```python
from build123d import *

# Parameters (mm, degrees)
SKETCH_R             = 1.6
SKETCH_R_2           = 6
PAD_DEPTH            = 4
SKETCH001_R          = 5
PAD001_DEPTH         = 12
SKETCH002_R          = 4.7
POCKET_DEPTH         = 13.001
SKETCH004_R          = 1.5
POCKET002_DEPTH      = 13.001
SKETCH005_R          = 1.5
POCKET003_DEPTH      = 4.001
POCKET003_DEPTH_BACK = 12.001
SKETCH006_R          = 4.7
SKETCH006_R_2        = 2.2
PAD002_DEPTH         = 6
SKETCH007_R          = 3
SKETCH007_R_2        = 1.5
PAD003_DEPTH         = 2
PAD003_DEPTH_BACK    = 2
SKETCH003_R          = 4.75
PAD004_DEPTH         = 2
SKETCH008_R          = 6.25
POCKET004_DEPTH      = 12.001
FILLET_R             = 1.5
FILLET001_R          = 3
FILLET002_R          = 1


with BuildPart() as part:
    # Sketch → Pad (new body)
    with BuildSketch(Plane.XY):
        Polygon((0, 20), (-26, 20), (-26, 0), (-26, -20), (0, -20), (20, -20), (20, 0), (20, 20), align=None)
        with Locations((-23, 5.9)):
            Circle(SKETCH_R, mode=Mode.SUBTRACT)
        with Locations((-23, -5.9)):
            Circle(SKETCH_R, mode=Mode.SUBTRACT)
        Circle(SKETCH_R_2, mode=Mode.SUBTRACT)
    extrude(amount=-PAD_DEPTH)

    # Sketch001 → Pad001 (join)
    with BuildSketch(Plane.XY):
        with Locations((13, -13)):
            Circle(SKETCH001_R)
        Polygon((0, 20), (20, 20), (20, 7), (0, 7), (-20, 7), (-20, 20), align=None)
    extrude(amount=PAD001_DEPTH)

    # Sketch002 (on DatumPlane) → Pocket (cut, through all)
    with BuildSketch(Plane.XZ.offset(-7)):
        with Locations((5.5, 5)):
            Circle(SKETCH002_R)
    extrude(amount=-POCKET_DEPTH, mode=Mode.SUBTRACT)

    # Sketch004 (on DatumPlane) → Pocket002 (cut, through all)
    with BuildSketch(Plane.XZ.offset(-7)):
        with Locations((-12, 5)):
            Circle(SKETCH004_R)
    extrude(amount=-POCKET002_DEPTH, mode=Mode.SUBTRACT)

    # Sketch005 → Pocket003 (cut, two sides)
    with BuildSketch(Plane.XY) as pocket003_sk:
        with Locations((13, -13)):
            Circle(SKETCH005_R)
        with Locations((13, 13)):
            Circle(SKETCH005_R)
    extrude(amount=-POCKET003_DEPTH, mode=Mode.SUBTRACT)
    extrude(pocket003_sk.sketch, amount=POCKET003_DEPTH_BACK, mode=Mode.SUBTRACT)

    # Sketch006 (on DatumPlane) → Pad002 (join)
    with BuildSketch(Plane.XZ.offset(-7)):
        with Locations((5.5, 5)):
            Circle(SKETCH006_R)
        with Locations((5.5, 5)):
            Circle(SKETCH006_R_2, mode=Mode.SUBTRACT)
    extrude(amount=-PAD002_DEPTH)

    # Sketch007 (on DatumPlane) → Pad003 (join, two sides)
    with BuildSketch(Plane.XZ.offset(-7)) as pad003_sk:
        with Locations((5.5, 5)):
            Circle(SKETCH007_R)
        with Locations((5.5, 5)):
            Circle(SKETCH007_R_2, mode=Mode.SUBTRACT)
    extrude(amount=PAD003_DEPTH)
    extrude(pad003_sk.sketch, amount=-PAD003_DEPTH_BACK)

    # Sketch003 (on DatumPlane) → Pad004 (join)
    with BuildSketch(Plane.XZ.offset(-7)):
        with BuildLine():
            ThreePointArc((-7.465411, 0), (-12, 11.75), (-16.534589, 0))
            Line((-16.534589, 0), (-7.465411, 0))
        make_face()
        with Locations((-12, 5)):
            Circle(SKETCH003_R, mode=Mode.SUBTRACT)
    extrude(amount=PAD004_DEPTH)

    # Sketch008 → Pocket004 (cut, through all)
    with BuildSketch(Plane.XY):
        Circle(SKETCH008_R)
    extrude(amount=POCKET004_DEPTH, mode=Mode.SUBTRACT)

    # Fillet
    fillet_edges = [part.edges().sort_by_distance(p)[0] for p in [
        (8, -13, 0),
    ]]
    fillet(fillet_edges, radius=FILLET_R)

    # Fillet001
    fillet001_edges = [part.edges().sort_by_distance(p)[0] for p in [
        (-26, -20, -2),
        (20, -20, -2),
        (20, 20, -2),
        (-26, 20, -2),
        (20, 7, 6),
        (-20, 20, 6),
    ]]
    fillet(fillet001_edges, radius=FILLET001_R)

    # Fillet002
    fillet002_edges = [part.edges().sort_by_distance(p)[0] for p in [
        (-20, 7, 6),
    ]]
    fillet(fillet002_edges, radius=FILLET002_R)


solid = part.part
```
Geometry: final body of the model. Coordinates: model frame, mm. A direction names the side the tool comes from. Coordinates: 2 decimals unless noted, no trailing zeros. Order: outer loops, then holes, each group sorted by start corner. A loop starts at its lowest first (then second) coordinate and runs counter-clockwise, first axis right, second up. Notation, with made-up numbers: (72.25, 38) - (119.25, 38) arc R8 cw to (119.25, 47) - close; hole circle Ø3 at (36.25, 78). An arc over 180 degrees is marked (long way). Write each question's results on one line, items separated by ' | '.
1) Section D-D, the plane x = 0. Return loops of the section in (y, z).
Results list:
outline: (-20, -4) - (-6, -4) - (-6, 0) - (-20, 0) - close; (6, -4) - (20, -4) - (20, 12) - (7, 12) - (7, 0) - (6, 0) - close
2) Section A-A, the plane x = 13. Return loops of the section in (y, z), plus the area to 3 significant figures.
Results list:
outline: (-20, -4) - (-14.5, -4) - (-14.5, 12) - (-18, 12) - (-18, 1.5) arc R1.5 cw to (-19.5, 0) - (-20, 0) - close; (-11.5, -4) - (11.5, -4) - (11.5, 12) - (7, 12) - (7, 0) - (-6.5, 0) arc R1.5 cw to (-8, 1.5) - (-8, 12) - (-11.5, 12) - close; (14.5, -4) - (20, -4) - (20, 12) - (14.5, 12) - close | area: 341 mm^2
3) Line query: line 1 (Y direction, x = 13, z = 6); line 2 (Y direction, x = 13, z = -3.1); line 3 (Y direction, x = -23, z = -2.15). Output: solid intervals per line, ascending. Write a range as from..to.
Results list:
line 1: -18..-14.5, -11.5..-8, 7..11.5, 14.5..20 | line 2: -20..-14.5, -11.5..11.5, 14.5..20 | line 3: -20..-7.5, -4.3..4.3, 7.5..20
4) Pin query (flat end, axial travel): pin 1 (2 mm diameter, centred on x = 5.5, y = -8, fed in from +Z); pin 2 (8 mm diameter, centred on x = -3, z = 8.5, fed in from -Y); pin 3 (5 mm diameter, centred on x = 7, z = 9.5, fed in from -Y). Return the tip coordinate at first contact, or that it passes through.
Results list:
pin 1: z = 0 | pin 2: y = 5 | pin 3: y = -16.57
5) Pull-direction query (Z, two-part tool) for faces 5 (the cylindrical face through (19.1, 19.14, 3.89)), 6 (the flat face through (-8, 0, -4)), 7 (the cylindrical face through (7.6, 10.97, 5.66)), 8 (the flat face through (11.8, -11.8, 12)); classes: pulls with the +Z half, pulls with the -Z half, needs draft (parallel to the pull), parting line crosses it, or undercut.
Results list:
face 5: needs draft | face 6: pulls with the -Z half | face 7: undercut | face 8: pulls with the +Z half
6) Section C-C, the plane z = 5. State how many separate pieces and enclosed holes the cut face has, plus the area to 3 significant figures.
Results list:
separate pieces: 4 | enclosed holes: 2 | area: 463 mm^2
7) Set-up query: faces 1 (the cylindrical face through (8.36, 6.01, 5.9)), 2 (the cylindrical face through (-15.5, 6.01, 8.21)), 3 (the flat face through (8, 13, 4)), 4 (the cylindrical face through (-19.14, 19.1, 6.08)). Return all of +Z, -Z, +X, -X, +Y, -Y with unobstructed straight access to the full face (end or side cutting, diameter ignored); none if empty.
Results list:
face 1: none | face 2: -Y | face 3: +Y | face 4: +Z, -X, +Y
8) Section B-B, the plane y = 0. Return loops of the section in (x, z), plus the area to 3 significant figures.
Results list:
outline: (-26, -4) - (-6, -4) - (-6, 0) - (-26, 0) - close; (6, -4) - (20, -4) - (20, 0) - (6, 0) - close | area: 136 mm^2
